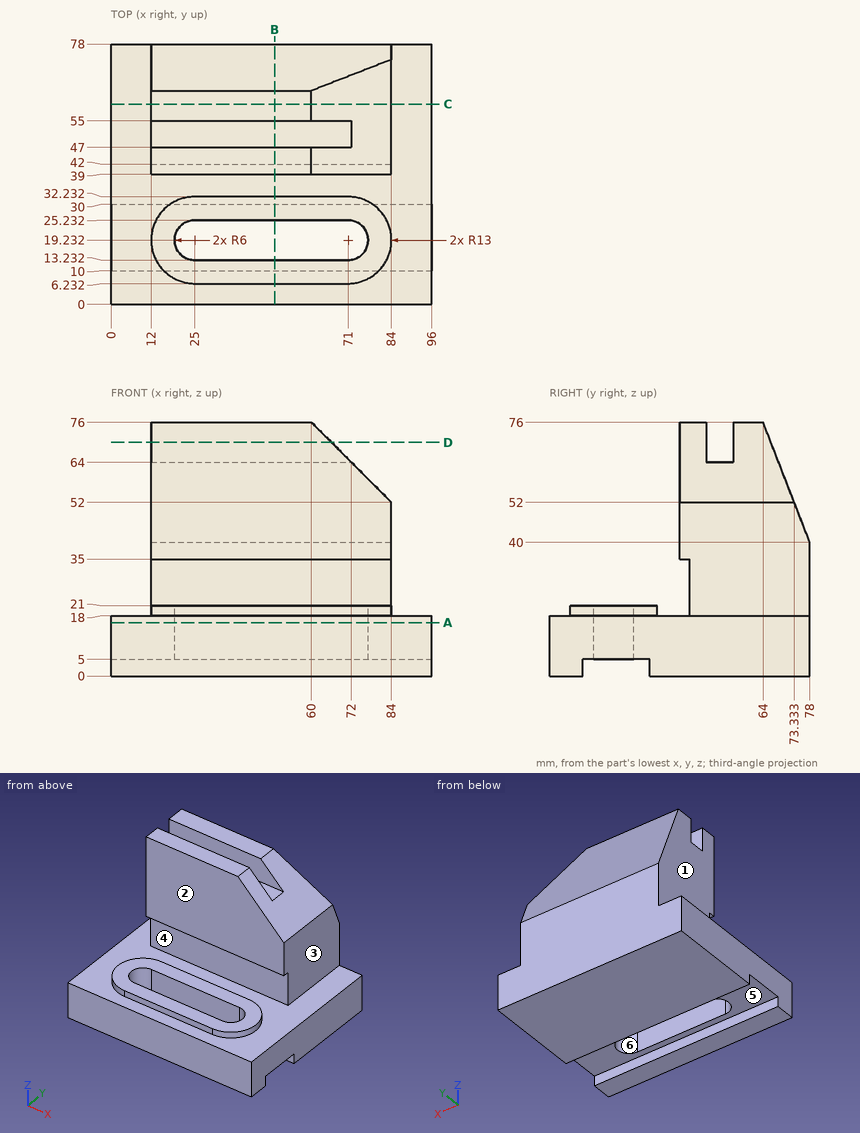
Answer from the drawing. Dimensions are ordinates in mm from the lowest x, y and z of the part. A direction names the side the tool comes from. Give positions to 0.01 mm unless a question says otherwise; leave off trailing zeros. Loops run counter-clockwise (first coordinate to the right, second up) from the corner with the lowest first, then second, coordinate; pieces in that order, holes last. Notation, with made-up numbers: (-25.75, 40) -> (20.25, 40) arc R21 cw to (20.25, 48) -> close; hole circle Ø3 at (56.25, -2). An arc over 180 degrees is marked (long way). One line per question, with ' | ' between items. Start each with the question number.
1) Each of these flat-tipped pins is pushed along its axis until it touches: pin 1 (8.5 mm diameter, centred on x = 66, z = 24.5, fed in from -Y); pin 2 (10 mm diameter, centred on y = 66, z = 42.5, fed in from +X); pin 3 (3.5 mm diameter, centred on x = 57, z = 67.5, fed in from -Y). Where does it stop, or does it pass through?
2) Section A-A, the plane z = 16 is taken. Determine the outline of the cut face in (x, y), then the cut area to 3 significant figures.
3) For the marked faces 1, 2 and 3, determine the directions among +Z, -Z, +X, -X, +Y, -Y from which every point of the face is accessible in a straight line to the end or side of a thin tool.
4) Determine the mould class of the marked faces 4, 5 and 6 for opening direction Z: +Z half, -Z half, draft (parallel to the pull), parting line (faces both ways), or undercut.
5) Section B-B, the plane x = 49 is taken. Determine the outline of the cut face in (y, z), then the cut area to 3 significant figures.
6) Section C-C, the plane y = 60 is taken. Determine the outline of the cut face in (x, z).
7) Section D-D, the plane z = 70 is taken. Determine the outline of the cut face in (x, y), then the cut area to 3 significant figures.
8) Straight lines are drawn through the part: L1, parallel to Y at x = 65, z = 7; L2, parallel to Y at x = 58.5, z = 27; L3, parallel to Y at x = 61.5, z = 39.5. For each, find the intervals that lie inside material, in ascending order.
Resolved:
1) pin 1: y = 6.23 | pin 2: x = 84 | pin 3: y = 39
2) outline: (0, 0) -> (96, 0) -> (96, 78) -> (0, 78) -> close; hole (25, 13.23) -> (71, 13.23) arc R6 ccw to (71, 25.23) -> (25, 25.23) arc R6 ccw to start | area: 6,820 mm2
3) face 1: +Z, -X, +Y, -Y | face 2: +Z, +X, -X, -Y | face 3: +Z, +X, +Y, -Y
4) face 4: undercut | face 5: -Z half | face 6: draft
5) outline: (0, 0) -> (10, 0) -> (10, 5) -> (13.23, 5) -> (13.23, 21) -> (6.23, 21) -> (6.23, 18) -> (0, 18) -> close; (25.23, 5) -> (30, 5) -> (30, 0) -> (78, 0) -> (78, 40) -> (64, 76) -> (55, 76) -> (55, 64) -> (47, 64) -> (47, 76) -> (39, 76) -> (39, 35) -> (42, 35) -> (42, 18) -> (32.23, 18) -> (32.23, 21) -> (25.23, 21) -> close | area: 3,050 mm2
6) outline: (0, 0) -> (96, 0) -> (96, 18) -> (84, 18) -> (84, 52) -> (60, 76) -> (12, 76) -> (12, 18) -> (0, 18) -> close
7) outline: (12, 39) -> (66, 39) -> (66, 47) -> (12, 47) -> close; (12, 55) -> (66, 55) -> (66, 66.33) -> (12, 66.33) -> close | area: 1,040 mm2
8) L1: 0 to 13.23, 25.23 to 78 | L2: 42 to 78 | L3: 39 to 78
